from build123d import *

# Parameters (mm, degrees)
F1_DEPTH = 12.7
F2_R     = 1.45
F3_DEPTH = 29.2862
F4_SIZE  = 1.27


with BuildPart() as f1:
    # F0 (on Top) → F1 (new body)
    with BuildSketch(Plane.XY):
        with BuildLine():
            Line((15, 2.625), (15, 8.975))
            Line((15, 8.975), (-15, 8.975))
            Line((-15, 8.975), (-15, -8.975))
            Line((-15, -8.975), (15, -8.975))
            Line((15, -8.975), (15, -2.625))
            Line((15, -2.625), (3.267087, -2.625))
            ThreePointArc((3.267087, -2.625), (-4.191, 0), (3.267087, 2.625))
            Line((3.267087, 2.625), (15, 2.625))
        make_face()
    extrude(amount=F1_DEPTH)

    # F2 (on face) → F3 (cut)
    with BuildSketch(Plane(origin=(0, 8.975, 0), x_dir=(-1, 0, 0), z_dir=(0, 1, 0))):
        with Locations((8.65, 6.35)):
            Circle(F2_R)
    extrude(amount=-F3_DEPTH, mode=Mode.SUBTRACT)

    # F4
    f4_edges = [f1.edges().sort_by_distance(p)[0] for p in [
        (-7.2, 8.975, 6.35),
        (-7.2, -8.975, 6.35),
    ]]
    chamfer(f4_edges, length=F4_SIZE)


solid = f1.part
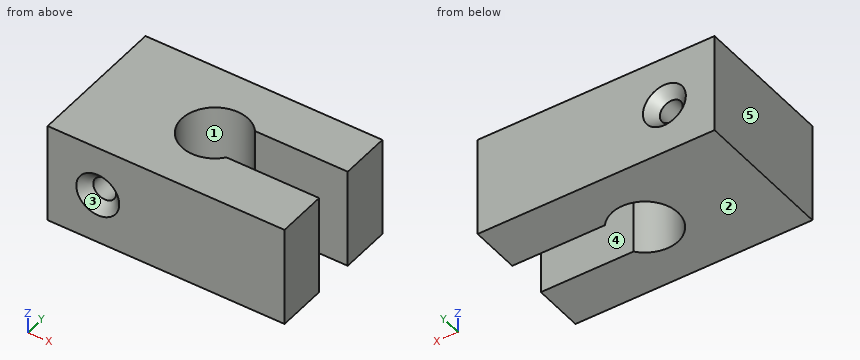
Geometry check sheet. Reference: the model listing, model coordinates, mm. Face numbers are marked on the shaded views. A direction names the side the tool comes from. Round coordinates to 2 decimals unless told otherwise and drop trailing zeros. Write each loop counter-clockwise with the first axis right and the second up, starting at its lowest first coordinate (ties: lowest second). Pieces come first, ordered by that corner, then holes. Notation, with made-up numbers: (79.25, -39.5) -> (122.25, -39.5) arc R17 cw to (122.25, -10.5) -> close; hole circle Ø2 at (-6, 47.25). An arc over 180 degrees is marked (long way). One line per item, written item: value. Start each with the question number.
(1) Draft check along Z on the marked faces 1, 2 and 3. Enter one of: +Z half, -Z half, draft (parallel to the pull), parting line (faces both ways), or undercut.
(2) Cross-section at C-C, the plane y = 5. Record the cut outline in (x, z).
(3) Go/stop test with a flat-tipped pin: pin 1 Ø2.5 at (x, z) = (-8.65, 6.35) entering from -Y. Record where the tip stops, or that it passes through.
(4) Scan lines: line 1 (Y direction, x = 0, z = 3) (3 decimals); line 2 (Z direction, x = -8.65, y = -1.5); line 3 (Y direction, x = 3.5, z = 6.5) (3 decimals). Record each from-to range of solid material in increasing order. Write a range as [from, to].
(5) Cross-section at B-B, the plane z = 6.35. Record the cut outline in (x, y) (3 decimals), and give its area (3 significant figures).
(6) Cross-section at D-D, the plane z = 12. Record the cut outline in (x, y) (3 decimals).
(7) Access from +Z, -Z, +X, -X, +Y, -Y to the whole of each face (thin tool, end or side, straight path). Record for the marked faces 4 and 5.
(8) Cross-section at A-A, the plane x = -8.65. Record the cut outline in (y, z) (3 decimals).
Answer:
1. face 1: draft
1. face 2: -Z half
1. face 3: undercut
2. outline: (-15, 0) -> (15, 0) -> (15, 12.7) -> (-15, 12.7) -> close; hole circle Ø2.9 at (-8.65, 6.35)
3. pin 1: through
4. line 1: [-8.975, -4.191], [4.191, 8.975]
4. line 2: [0, 4.9], [7.8, 12.7]
4. line 3: [-8.975, -2.625], [2.625, 8.975]
5. outline: (-15, -8.975) -> (-11.37, -8.975) -> (-10.1, -7.705) -> (-10.1, 7.705) -> (-11.37, 8.975) -> (-15, 8.975) -> close; (-7.2, -7.705) -> (-5.93, -8.975) -> (15, -8.975) -> (15, -2.625) -> (3.267, -2.625) arc R4.191 cw (long way) to (3.267, 2.625) -> (15, 2.625) -> (15, 8.975) -> (-5.93, 8.975) -> (-7.2, 7.705) -> close
5. area: 370 mm²
6. outline: (-15, -8.975) -> (15, -8.975) -> (15, -2.625) -> (3.267, -2.625) arc R4.191 cw (long way) to (3.267, 2.625) -> (15, 2.625) -> (15, 8.975) -> (-15, 8.975) -> close
7. face 4: +Z, -Z, +X
7. face 5: +Z, -Z, -X, +Y, -Y
8. outline: (-8.975, 0) -> (8.975, 0) -> (8.975, 3.63) -> (7.705, 4.9) -> (-7.705, 4.9) -> (-8.975, 3.63) -> close; (-8.975, 9.07) -> (-7.705, 7.8) -> (7.705, 7.8) -> (8.975, 9.07) -> (8.975, 12.7) -> (-8.975, 12.7) -> close
